Study the drawing (mm; zero at the part's minimum x, y, z) and answer. Give positions to 0.01 mm unless a question says otherwise; leave off trailing zeros. Write each loop counter-clockwise with the first axis right and the second up, starting at its lowest first coordinate (ties: lowest second). Pieces come first, ordered by that corner, then holes. Notation, with made-up numbers: M 82.5,39.25 L 131.5,39.25 A8 ccw 131.5,51.25 Z; hole C 65,43.25 d10. An arc over 180 degrees is marked long. Use a Markdown table: item, result. Add a question column.
Item 1: A cutting plane is placed at C-C on z = 1.55. Determine the outline of the cut face in (x, y).
Item 2: Given P1, Ø1.5, axis at y = 4, z = 2, coming from the +X side; P2, Ø1, axis at y = 3.5, z = 2, coming from the -X side; P3, Ø1, axis at x = 5, z = 1.5, coming from the +Y side, each flat-ended and moving along its own axis, determine where each tip first touches the part or whether it passes through.
Item 3: Consider probe 1 along Y at (x, z) = (6, 2.7); probe 2 along Y at (x, z) = (8, 0.5); probe 3 along X at (y, z) = (7.5, 1.2). Determine where each line is inside the solid, lowest interval first. Write a range as [from, to].
Item 4: A cutting plane is placed at A-A on y = 6. Determine the outline of the cut face in (x, z).
Item 5: The mould has two halves that part along Y. Classify the marked faces 1, 2 and 3: pulls with the +Y half, pulls with the -Y half, needs draft (parallel to the pull), parting line crosses it, or undercut.
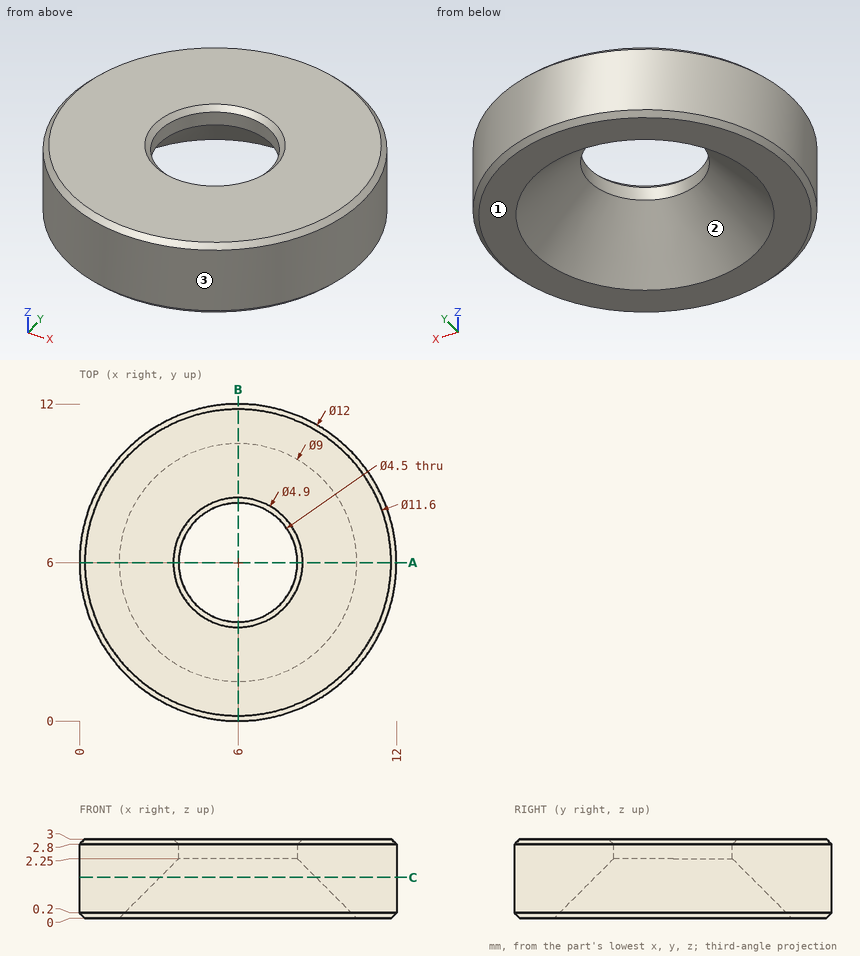
Filled in:
| question | item | result |
|---|---|---|
| 1 | outline | C 6,6 d12; hole C 6,6 d5.9 |
| 2 | P1 | x = 11.87 |
| 2 | P2 | x = 0.34 |
| 2 | P3 | y = 11.98 |
| 3 | probe 1 | [0, 3.75], [8.25, 12] |
| 3 | probe 2 | [0.34, 2.54], [9.46, 11.66] |
| 3 | probe 3 | [0.19, 3.06], [8.94, 11.81] |
| 4 | outline | M 0,0.2 L 0.2,0 L 1.5,0 L 3.75,2.25 L 3.75,2.8 L 3.55,3 L 0.2,3 L 0,2.8 Z; M 8.25,2.25 L 10.5,0 L 11.8,0 L 12,0.2 L 12,2.8 L 11.8,3 L 8.45,3 L 8.25,2.8 Z |
| 5 | face 1 | needs draft |
| 5 | face 2 | undercut |
| 5 | face 3 | parting line crosses it |
